Source: CAD feature listing. Evaluate the final solid. Frame: model axes, mm. Face numbers are marked on the shaded views. Give positions to 0.01 mm unless a question says otherwise; leave off trailing zeros. Write each loop counter-clockwise with the first axis right and the second up, starting at its lowest first coordinate (ties: lowest second). Pieces come first, ordered by that corner, then holes. Notation, with made-up numbers: (48, -3) - (54, -3) arc R16 cw to (54, 2) - close; hole circle Ø4 at (57.5, 19). An arc over 180 degrees is marked (long way). Answer as a JSON object with one key per item and string values. Group by question number.
from build123d import *

# Parameters (mm, degrees)
BOSS_EXTRUDE1_DEPTH      = 10
BOSS_EXTRUDE1_DEPTH_BACK = 15
SKETCH1_R                = 55
SKETCH1_R_2              = 25
SKETCH2_R                = 50
SKETCH2_R_2              = 47
SKETCH2_R_3              = 4.75
CUT_EXTRUDE1_DEPTH       = 15


with BuildPart() as part:
    # Sketch1 → Boss-Extrude1 (new, two sides: drawn at the far end of the back side and taken through both)
    with BuildSketch(Plane.XY.offset(-BOSS_EXTRUDE1_DEPTH_BACK)):
        Circle(SKETCH1_R)
        Circle(SKETCH1_R_2, mode=Mode.SUBTRACT)
    extrude(amount=BOSS_EXTRUDE1_DEPTH + BOSS_EXTRUDE1_DEPTH_BACK)

    # Sketch2 → Cut-Extrude1 (cut)
    # profile 1 of 3: a face of its own
    with BuildSketch(Plane.XY.offset(10)):
        Circle(SKETCH2_R)
        Circle(SKETCH2_R_2, mode=Mode.SUBTRACT)
    # profile 2 of 3: a face of its own
    with BuildSketch(Plane.XY.offset(10)):
        with Locations((-34.5, 0)):
            Circle(SKETCH2_R_3)
    # profile 3 of 3: a face of its own
    with BuildSketch(Plane.XY.offset(10)):
        with Locations((34.5, 0)):
            Circle(SKETCH2_R_3)
    extrude(amount=-CUT_EXTRUDE1_DEPTH, mode=Mode.SUBTRACT)


solid = part.part
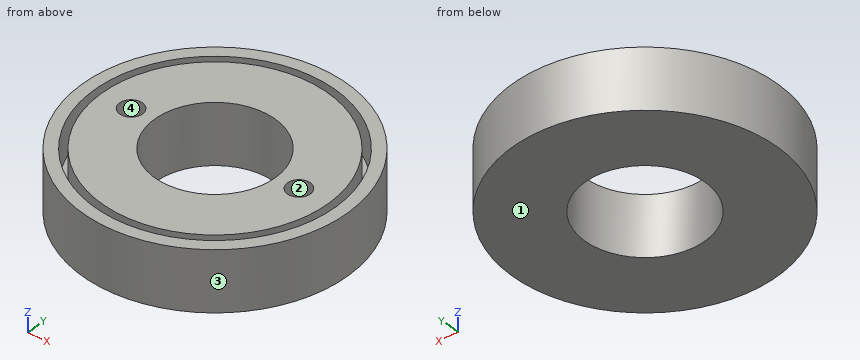
Q1. Section C-C on z = 1.25. Return the cut outline in (x, y), then the cut area to 3 significant figures.
Q2. Draft query along X for the marked faces 1, 2, 3 and 4. Return one class per face: released by +X, released by -X, zero draft, split by the parting line, or undercut.
Q3. Ray query, probe 1 along Y at (x, z) = (0, 0.25); probe 2 along Y at (x, z) = (34.5, 0.75); probe 3 along X at (y, z) = (-12, -0.75). Return the intervals inside material, ascending. Write a range as [from, to].
Q4. Section D-D on x = 18. Return the cut outline in (y, z), then the cut area to 3 significant figures.
Q5. First-contact query: pin 1 Ø1.5 at (x, z) = (1.5, -5.5) entering from +Y; pin 2 Ø8 at (y, z) = (32.5, -8.5) entering from -X; pin 3 Ø2 at (y, z) = (10, 6.5) entering from -X. Flat tips, straight axial feed; report the tip coordinate or a pass-through.
Q6. Section A-A on x = 0. Return the cut outline in (y, z), then the cut area to 3 significant figures.
Q7. Section B-B on y = 0. Return the cut outline in (x, z).
Taken from the geometry:
{
 "1": {"outline": "circle Ø110 at (0, 0); circle Ø94 at (0, 0); hole circle Ø100 at (0, 0); hole circle Ø9.5 at (-34.5, 0); hole circle Ø50 at (0, 0); hole circle Ø9.5 at (34.5, 0)", "area": "6,480 mm²"},
 "2": {"face 1": "zero draft", "face 2": "undercut", "face 3": "split by the parting line", "face 4": "undercut"},
 "3": {"probe 1": "y = [-55, -50], [-47, -25], [25, 47], [50, 55]", "probe 2": "y = [-42.83, -36.19], [-31.92, -4.75], [4.75, 31.92], [36.19, 42.83]", "probe 3": "x = [-53.67, -48.54], [-45.44, -21.93], [21.93, 45.44], [48.54, 53.67]"},
 "4": {"outline": "(-51.97, -15) - (-17.35, -15) - (-17.35, 10) - (-43.42, 10) - (-43.42, -5) - (-46.65, -5) - (-46.65, 10) - (-51.97, 10) - close; (17.35, -15) - (51.97, -15) - (51.97, 10) - (46.65, 10) - (46.65, -5) - (43.42, -5) - (43.42, 10) - (17.35, 10) - close", "area": "1,630 mm²"},
 "5": {"pin 1": "stops at y = 54.99", "pin 2": "stops at x = -47.04", "pin 3": "stops at x = -54.26"},
 "6": {"outline": "(-55, -15) - (-25, -15) - (-25, 10) - (-47, 10) - (-47, -5) - (-50, -5) - (-50, 10) - (-55, 10) - close; (25, -15) - (55, -15) - (55, 10) - (50, 10) - (50, -5) - (47, -5) - (47, 10) - (25, 10) - close", "area": "1,410 mm²"},
 "7": {"outline": "(-55, -15) - (-25, -15) - (-25, 10) - (-29.75, 10) - (-29.75, -5) - (-39.25, -5) - (-39.25, 10) - (-47, 10) - (-47, -5) - (-50, -5) - (-50, 10) - (-55, 10) - close; (25, -15) - (55, -15) - (55, 10) - (50, 10) - (50, -5) - (47, -5) - (47, 10) - (39.25, 10) - (39.25, -5) - (29.75, -5) - (29.75, 10) - (25, 10) - close"}
}
